Input: part model. Units: mm. Frame: model coordinates. A direction names the side the tool comes from. Coordinates: 2 decimals unless noted, no trailing zeros. Write each loop counter-clockwise with the first axis right and the second up, starting at its lowest first coordinate (ties: lowest second). Pieces come first, ordered by that corner, then holes. Notation, with made-up numbers: (-2.5, 74.5) - (19.5, 74.5) arc R34 cw to (19.5, 109.5) - close; hole circle Ø6 at (-18, -5.75). An arc over 180 degrees is marked (long way). One line per question, with ' | ' between items. Start each with the question number.
1) First-contact query: P1, Ø2.5, axis at x = 8.21, y = 4.55, coming from the +Z side; P2, Ø6, axis at x = 10.5, z = -5.5, coming from the +Y side; P3, Ø4, axis at x = 12.5, z = -1.5, coming from the +Y side; P4, Ø6, axis at y = 7.5, z = -7.5, coming from the +X side. Flat tips, straight axial feed; report the tip coordinate or a pass-through.
2) Section query A-A on x = 9.25. Return loops of the section in (y, z).
3) Draft query along Z for faces 3 (the flat face through (4, 6, 2)), 4 (the cylindrical face through (1.64, 1.01, -9.4)), 5 (the flat face through (9, 1, -6)), 6 (the cylindrical face through (-0.99, 5.56, -7.1)). Return one class per face: released by +Z, released by -Z, zero draft, split by the parting line, or undercut.
4) Line query: line 1 (Y direction, x = 5.5, z = -6.75); line 2 (X direction, y = 12.25, z = -2). Output: solid intervals per line, ascending.
5) Section query C-C on x = 0.75. Return loops of the section in (y, z).
6) Section query D-D on y = 4.25. Return loops of the section in (x, z).
7) Section query B-B on z = -0.5. Return loops of the section in (x, y).
8) Reachability of faces 1 (the flat face through (4, 2, -5)), 2 (the cylindrical face through (9.706, 4.616, 0.986)) from +Z, -Z, +X, -X, +Y, -Y: full face, straight path, thin tool, end or side. Return the list, or none.
```python
from build123d import *

# Parameters (mm, degrees)
BOSS_EXTRUDE1_DEPTH      = 2
BOSS_EXTRUDE2_DEPTH      = 15
BOSS_EXTRUDE2_DEPTH_BACK = 2
CUT_EXTRUDE1_DEPTH       = 15
CUT_EXTRUDE2_DEPTH       = 15
SKETCH5_R                = 1.5
CUT_EXTRUDE3_DEPTH       = 15
SKETCH6_R                = 1.5
CUT_EXTRUDE4_DEPTH       = 15
SKETCH7_R                = 1.5
CUT_EXTRUDE5_DEPTH       = 15
IZIM1_W                  = 17
IZIM1_H                  = 17
KES_EKSTR_ZYON1_DEPTH    = 3


with BuildPart() as part:
    # Sketch1 → Boss-Extrude1 (new body)
    with BuildSketch(Plane(origin=(0, 0, 0), x_dir=(1, 0, 0), z_dir=(0, 1, 0))):
        Polygon((0, 15), (15, 0), (0, 0), align=None)
    extrude(amount=BOSS_EXTRUDE1_DEPTH)

    # Sketch2 → Boss-Extrude2 (add, two sides: drawn at the far end of the back side and taken through both)
    with BuildSketch(Plane(origin=(0, 2, 0), x_dir=(1, 0, 0), z_dir=(0, 1, 0)).offset(-BOSS_EXTRUDE2_DEPTH_BACK)):
        Polygon((-2, -2), (15, -2), (15, 0), (0, 0), (0, 15), (-2, 15), align=None)
    extrude(amount=BOSS_EXTRUDE2_DEPTH + BOSS_EXTRUDE2_DEPTH_BACK)

    # Sketch3 → Cut-Extrude1 (cut)
    with BuildSketch(Plane(origin=(0, 0, 0), x_dir=(0, 0, -1), z_dir=(1, 0, 0))):
        Polygon((15, 2), (0, 17), (15, 17), align=None)
    extrude(amount=-CUT_EXTRUDE1_DEPTH, mode=Mode.SUBTRACT)

    # Sketch4 → Cut-Extrude2 (cut)
    with BuildSketch(Plane(origin=(0, 0, 0), x_dir=(-1, 0, 0), z_dir=(0, 0, -1))):
        Polygon((0, 17), (-15, 2), (-15, 17), align=None)
    extrude(amount=-CUT_EXTRUDE2_DEPTH, mode=Mode.SUBTRACT)

    # Sketch5 → Cut-Extrude3 (cut)
    with BuildSketch(Plane(origin=(0, 0, 0), x_dir=(0, 0, -1), z_dir=(1, 0, 0))):
        with Locations((2.550252532, 10.207106781)):
            Circle(SKETCH5_R)
        with Locations((8.207106781, 4.550252532)):
            Circle(SKETCH5_R)
    extrude(amount=-CUT_EXTRUDE3_DEPTH, mode=Mode.SUBTRACT)

    # Sketch6 → Cut-Extrude4 (cut)
    with BuildSketch(Plane(origin=(0, 0, 0), x_dir=(-1, 0, 0), z_dir=(0, 0, -1))):
        with Locations((-2.550252532, 10.207106781)):
            Circle(SKETCH6_R)
        with Locations((-8.207106781, 4.550252532)):
            Circle(SKETCH6_R)
    extrude(amount=-CUT_EXTRUDE4_DEPTH, mode=Mode.SUBTRACT)

    # Sketch7 → Cut-Extrude5 (cut)
    with BuildSketch(Plane(origin=(0, 2, 0), x_dir=(1, 0, 0), z_dir=(0, 1, 0))):
        with Locations(Location((2.550252532, 8.207106781, 0), (0, 0, 270))):
            Circle(SKETCH7_R)
        with Locations(Location((8.207106781, 2.550252532, 0), (0, 0, 270))):
            Circle(SKETCH7_R)
    extrude(amount=-CUT_EXTRUDE5_DEPTH, mode=Mode.SUBTRACT)

    # Çizim1 → Kes-Ekstrüzyon1 (cut)
    with BuildSketch(Plane(origin=(0, 0, -15), x_dir=(-1, 0, 0), z_dir=(0, 0, -1))):
        with Locations((-6.5, 8.5)):
            Rectangle(IZIM1_W, IZIM1_H)
    extrude(amount=-KES_EKSTR_ZYON1_DEPTH, mode=Mode.SUBTRACT)


solid = part.part
```
Answer key:
1) P1: through | P2: y = 2 | P3: y = 5.82 | P4: x = 0
2) outline: (0, -5.75) - (2, -5.75) - (2, -3.63) - (0, -3.63) - close; (0, -1.47) - (2, -1.47) - (2, 0) - (3.47, 0) - (3.47, 2) - (0, 2) - close; (5.63, 0) - (7.75, 0) - (7.75, 2) - (5.63, 2) - close
3) face 3: released by +Z | face 4: undercut | face 5: released by -Z | face 6: undercut
4) line 1: 0 to 2 | line 2: -2 to 0
5) outline: (0, -12) - (2, -12) - (2, 0) - (16.25, 0) - (16.25, 2) - (0, 2) - close
6) outline: (-2, -12) - (0, -12) - (0, -9.68) - (-2, -9.68) - close; (-2, -6.74) - (0, -6.74) - (0, 0) - (6.74, 0) - (6.74, 2) - (-2, 2) - close; (9.68, 0) - (12.75, 0) - (12.75, 2) - (9.68, 2) - close
7) outline: (-2, 0) - (14.5, 0) - (14.5, 2) - (0, 2) - (0, 16.5) - (-2, 16.5) - close
8) face 1: -Z, +X, +Y | face 2: +Z, -Z
